Could you check a few things on this model? Use its own coordinates, in mm. A direction names the side the tool comes from. Round coordinates to 2 decimals unless told otherwise and drop trailing zeros. Order: outer loops, then holes, each group sorted by start corner. A loop starts at its lowest first (then second) coordinate and runs counter-clockwise, first axis right, second up. Notation, with made-up numbers: (58.5, -20) - (109.5, -20) arc R18 ccw to (109.5, -8) - close; hole circle Ø4 at (65, 40). An arc over 180 degrees is marked (long way). Return JSON: item names as keys, results as strings. Group by question number.
Autodesk Inventor part; units mm, degrees
ref_plane "YZ Plane" through (0, 0, 0) normal (1, 0, 0) x (0, 1, 0)
ref_plane "XZ Plane" through (0, 0, 0) normal (0, 1, 0) x (-1, 0, 0)
ref_plane "XY Plane" through (0, 0, 0) normal (0, 0, 1) x (1, 0, 0)
sketch "Sketch1" plane through (0, 0, 0) normal (0, 0, 1) x (1, 0, 0)
  line L0 (0, 0) -> (58, 0)
  line L1 (58, 0) -> (58, 120)
  line L2 (58, 120) -> (0, 120)
  line L3 (0, 120) -> (0, 0)
  line L4 (58, 115) -> (81, 115)
  line L5 (81, 115) -> (81, 5)
  line L6 (81, 5) -> (58, 5)
  line L7 (58, 5) -> (58, 115)
  line L8 (0, 115) -> (-23, 115)
  line L9 (-23, 115) -> (-23, 5)
  line L10 (-23, 5) -> (0, 5)
  line L11 (0, 5) -> (0, 115)
  point P0 (0, 5)
  dimension "d0" = 58
  dimension "d1" = 120
  dimension "d20" = 23
  dimension "d21" = 5
  dimension "d22" = 5
  dimension "d26" = 23
  dimension "d27" = 5
  dimension "d28" = 5
extrude "Extrusion1" add sketch "Sketch1" along normal blind 2
sketch "Sketch2" plane through (0, 0, 2) normal (0, 0, 1) x (1, 0, 0)
  line L0 (58, 120) -> (0, 120)
  line L1 (58, 0) -> (58, 120)
  line L2 (0, 120) -> (58, 120)
  line L3 (58, 120) -> (58, 0)
  line L4 (58, 0) -> (0, 0)
  line L5 (0, 0) -> (0, 120)
  line L6 (2, 118) -> (56, 118)
  line L7 (56, 118) -> (56, 2)
  line L8 (56, 2) -> (2, 2)
  line L9 (2, 2) -> (2, 118)
  line L10 (-23, 115) -> (-23, 5)
  line L11 (-23, 115) -> (2, 115)
  line L12 (2, 115) -> (2, 55.5525)
  line L13 (-23, 5) -> (-23, 115)
  line L14 (-21, 113) -> (2, 113)
  line L15 (0, 113) -> (0, 57.5525)
  line L16 (-21, 7) -> (-21, 113)
  line L17 (-21, 7) -> (2, 7)
  line L18 (-23, 5) -> (0, 5)
  line L19 (-23, 5) -> (2, 5)
  line L20 (81, 115) -> (58, 115)
  line L21 (58, 115) -> (81, 115)
  line L22 (81, 115) -> (81, 5)
  line L23 (58, 5) -> (81, 5)
  line L24 (81, 5) -> (58, 5)
  line L25 (56, 7) -> (79, 7)
  line L26 (79, 7) -> (79, 113)
  line L27 (79, 113) -> (56, 113)
  point P0 (0, 0)
  point P1 (0, 115)
  point P2 (2, 113)
  point P3 (2, 7)
  dimension "d4" = 2
  dimension "d5" = 2
  dimension "d6" = 2
  dimension "d7" = 2
  dimension "d30" = 2
  dimension "d31" = 2
  dimension "d32" = 2
  dimension "d33" = 2
  dimension "d34" = 2
  dimension "d35" = 2
extrude "Extrusion2" add sketch "Sketch2" along normal blind 15 contours L1 L27 L7 L6 L9 L11 L5 L0 | L20 L22 L23 L1 L25 L26 L27 | L11 L9 L14 L5 | L5 L14 L16 L17 L18 L10 L11 | L1 L4 L5 L19 L9 L8 L7 L25 | L17 L9 L19 L5
sketch "Sketch6" plane through (0, 120, 0) normal (0, 1, 0) x (1, 0, 0)
  circle A0 centre (29, -8.5) radius 6
  circle A1 centre (39, -8.5) radius 1.5
  circle A2 centre (19, -8.5) radius 1.5
  line L0 (58, 0) -> (0, 0)
  line L1 (58, 0) -> (58, -17)
  line L2 (0, 0) -> (0, -17)
  dimension "d46" = 12
  dimension "d47" = 3
  dimension "d48" = 3
  dimension "d49" = 10
  dimension "d50" = 10
  dimension "d51" = 8.5
  dimension "d52" = 8.5
  dimension "d53" = 8.5
  dimension "d54" = 58
  dimension "d55" = 29
extrude "Extrusion4" cut sketch "Sketch6" against normal up to surface (120 mm away)
equation "\"d52\" = d51"
equation "\"d53\" = d51"
equation "\"d55\" = 0.5 * d54"
properties part number "corpo2"
1) For faces 4 (the flat face through (-10, 113, 9)), 5 (the flat face through (28, 61, 0)), 6 (the flat face through (22, 0, 8)), 7 (the flat face through (69, 115, 8)), 8 (the flat face through (58, 2, 8)), which set-ups out of +Z, -Z, +X, -X, +Y, -Y let a thin tool reach every point of the face, with its end or its side?
2) We'd pull the mould along Y, two halves only. Please class faces 1 (the flat face through (0, 118, 8)), 2 (the flat face through (70, 5, 8)), 3 (the flat face through (2, 4, 9)): +Y half, -Y half, draft (parallel to the pull), parting line (faces both ways), or undercut.
3) Will these pins go through, and if not, where does the flat tip stop? pin 1 (7.5 mm diameter, centred on x = 70.5, z = 10, fed in from -Y); pin 2 (1.8 mm diameter, centred on x = 19, z = 8.5, fed in from -Y); pin 3 (5 mm diameter, centred on x = 69.5, z = 11.5, fed in from +Y); pin 4 (3 mm diameter, centred on x = -9.5, y = 75, fed in from +Z).
4) If I drill on line 1 along X through (y, z) = (119.45, 8.5); line 2 along Y through (x, z) = (69, 12); line 3 along X through (y, z) = (16, 10.75), over which ranges is the centre line in solid material (lowest first)? Write a range as from..to.
5) I want a section at A-A, the plane x = 29. List the corners of the cut face in (y, z) for me.
6) I want a section at D-D, the plane y = 40. List the corners of the cut face in (x, z) for me, plus the area to 3 significant figures.
7) I want a section at C-C, the plane x = 66.5. List the corners of the cut face in (y, z) for me, plus the area to 3 significant figures.
Outcome:
{
 "1": {"face 4": "+Z", "face 5": "-Z, +X, -X, +Y, -Y", "face 6": "+Z, -Z, +X, -X, -Y", "face 7": "+Z, -Z, +X, +Y", "face 8": "+Z, -Z, +X, -Y"},
 "2": {"face 1": "draft", "face 2": "-Y half", "face 3": "undercut"},
 "3": {"pin 1": "y = 5", "pin 2": "through", "pin 3": "y = 115", "pin 4": "z = 2"},
 "4": {"line 1": "0..17.5, 20.5..23, 35..37.5, 40.5..58", "line 2": "5..7, 113..115", "line 3": "-23..-21, 79..81"},
 "5": {"outline": "(0, 0) - (120, 0) - (120, 2.5) - (118, 2.5) - (118, 2) - (2, 2) - (2, 2.5) - (0, 2.5) - close; (0, 14.5) - (2, 14.5) - (2, 17) - (0, 17) - close; (118, 14.5) - (120, 14.5) - (120, 17) - (118, 17) - close"},
 "6": {"outline": "(-23, 0) - (81, 0) - (81, 17) - (79, 17) - (79, 2) - (-21, 2) - (-21, 17) - (-23, 17) - close", "area": "268 mm^2"},
 "7": {"outline": "(5, 0) - (115, 0) - (115, 17) - (113, 17) - (113, 2) - (7, 2) - (7, 17) - (5, 17) - close", "area": "280 mm^2"}
}
